Can you work these out from the model? Positions are in its coordinate system, mm. Face numbers are marked on the shaded views. Give positions to 0.01 mm unless a question says otherwise; leave off trailing zeros. Write each loop counter-clockwise with the first axis right and the second up, starting at its lowest first coordinate (ties: lowest second). Pieces come first, ordered by that corner, then holes.
from build123d import *

# Parameters (mm, degrees)
ESQUISSE1_R                  = 12
ESQUISSE1_R_2                = 10
BOSS_EXTRU_1_DEPTH           = 21
ESQUISSE2_R                  = 12
BOSS_EXTRU_2_DEPTH           = 24
ENL_V_MAT_EXTRU_1_DEPTH      = 49.093658626
ENL_V_MAT_EXTRU_1_DEPTH_BACK = 49.093658626
ENL_V_MAT_EXTRU_2_DEPTH      = 49.246865329
ENL_V_MAT_EXTRU_2_DEPTH_BACK = 49.246865329
ESQUISSE4_R                  = 1.65


with BuildPart() as part:
    # Esquisse1 → Boss.-Extru.1 (new body)
    with BuildSketch(Plane.XY):
        with Locations(Location((0, 0, 0), (0, 0, 180))):
            Circle(ESQUISSE1_R)
        with Locations(Location((0, 0, 0), (0, 0, 180))):
            Circle(ESQUISSE1_R_2, mode=Mode.SUBTRACT)
    extrude(amount=BOSS_EXTRU_1_DEPTH)

    # Esquisse2 → Boss.-Extru.2 (add)
    with BuildSketch(Plane.XY.offset(21)):
        with Locations(Location((0, 0, 0), (0, 0, 180))):
            Circle(ESQUISSE2_R)
    extrude(amount=BOSS_EXTRU_2_DEPTH)

    # Esquisse3 → Enlèv. mat.-Extru.1 (cut, two sides: drawn at the far end of the back side and taken through both)
    with BuildSketch(Plane(origin=(0, 0, 0), x_dir=(0, 0, -1), z_dir=(1, 0, 0)).offset(-ENL_V_MAT_EXTRU_1_DEPTH_BACK)):
        with BuildLine():
            Line((-33, 12), (-45, 12))
            Line((-45, 12), (-50, 0))
            Line((-50, 0), (-45, -12))
            Line((-45, -12), (-33, -12))
            ThreePointArc((-33, -12), (-45, 0), (-33, 12))
        make_face()
        with BuildLine():
            Line((-23.018016229, 0.6), (0, 0.6))
            Line((0, 0.6), (0, -0.6))
            Line((0, -0.6), (-23.018016229, -0.6))
            ThreePointArc((-23.018016229, -0.6), (-43, 0), (-23.018016229, 0.6))
        make_face()
    extrude(amount=ENL_V_MAT_EXTRU_1_DEPTH + ENL_V_MAT_EXTRU_1_DEPTH_BACK, mode=Mode.SUBTRACT)

    # Esquisse4 → Enlèv. mat.-Extru.2 (cut, two sides: drawn at the far end of the back side and taken through both)
    with BuildSketch(Plane(origin=(0, -0.6, 0), x_dir=(1, 0, 0), z_dir=(0, 1, 0)).offset(-ENL_V_MAT_EXTRU_2_DEPTH_BACK)):
        with Locations(Location((0, -16, 0), (0, 0, 270))):
            Circle(ESQUISSE4_R)
        with Locations(Location((0, -5, 0), (0, 0, 270))):
            Circle(ESQUISSE4_R)
    extrude(amount=ENL_V_MAT_EXTRU_2_DEPTH + ENL_V_MAT_EXTRU_2_DEPTH_BACK, mode=Mode.SUBTRACT)


solid = part.part
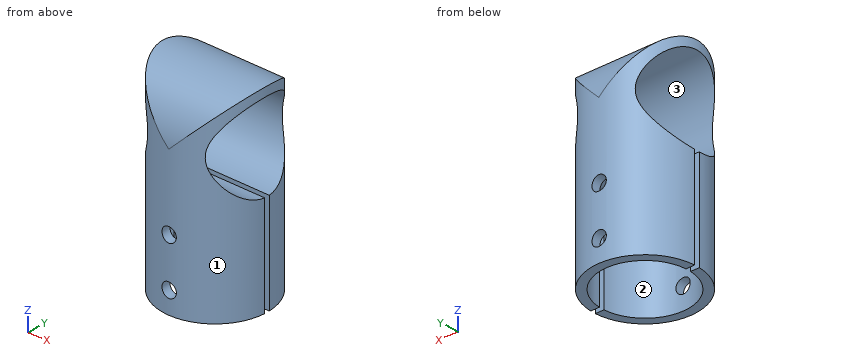
(1) Will these pins go through, and if not, where does the flat tip stop? P1, Ø5.5, axis at x = 0, z = 16, coming from the +Y side; P2, Ø4.5, axis at x = -2, y = -6, coming from the -Z side; P3, Ø1.5, axis at y = -7, z = 21.5, coming from the -X side; P4, Ø1, axis at x = 7, y = 5.5, coming from the +Z side.
Returned:
P1: stops at y = 12
P2: stops at z = 21
P3: stops at x = -10.24
P4: stops at z = 43.91
(2) If we mould it in two halves opening along X, with no side actions, what happens to the marked faces 1, 2 and 3? For each: +X half, -X half, draft (parallel to the pull), parting line (faces both ways), or undercut.
Returned:
face 1: parting line
face 2: undercut
face 3: draft
(3) Imagine slicing it at A-A, the plane x = 0. Write out the boundary of the cut face in (y, z).
Returned:
outline: (-12, 0) - (-10, 0) - (-10, 3.35) - (-12, 3.35) - close; (-12, 6.65) - (-10, 6.65) - (-10, 14.35) - (-12, 14.35) - close; (-12, 17.65) - (-10, 17.65) - (-10, 21) - (-0.6, 21) - (-0.6, 23.02) arc R10 cw (long way) to (0.6, 23.02) - (0.6, 21) - (10, 21) - (10, 17.65) - (12, 17.65) - (12, 33) arc R12 ccw to (-12, 33) - close; (10, 0) - (12, 0) - (12, 3.35) - (10, 3.35) - close; (10, 6.65) - (12, 6.65) - (12, 14.35) - (10, 14.35) - close
(4) Imagine slicing it at B-B, the plane y = 7.25. Write out the boundary of the cut face in (x, z), plus the area to 3 significant figures.
Returned:
outline: (-9.56, 0) - (-6.89, 0) - (-6.89, 21) - (6.89, 21) - (6.89, 0) - (9.56, 0) - (9.56, 26.11) - (-9.56, 26.11) - close; (-9.56, 39.89) - (9.56, 39.89) - (9.56, 42.56) - (-9.56, 42.56) - close
area: 261 mm2
(5) Imagine slicing it at C-C, the plane z = 16. Write out the boundary of the cut face in (x, y) (3 decimals).
Returned:
outline: (-11.985, -0.6) arc R12 ccw to (-1.65, -11.886) - (-1.65, -9.863) arc R10 cw to (-9.982, -0.6) - close; (-11.985, 0.6) - (-9.982, 0.6) arc R10 cw to (-1.65, 9.863) - (-1.65, 11.886) arc R12 ccw to start; (1.65, -11.886) arc R12 ccw to (11.985, -0.6) - (9.982, -0.6) arc R10 cw to (1.65, -9.863) - close; (1.65, 9.863) arc R10 cw to (9.982, 0.6) - (11.985, 0.6) arc R12 ccw to (1.65, 11.886) - close
(6) If I drill on L1, parallel to Z at x = -0.5, y = -10.75; L2, parallel to Z at x = 0, y = -11.05; L3, parallel to Z at x = 5, y = -5.5, over which ranges is the centre line in solid material (lowest first)?
Returned:
L1: z = 0 to 3.43, 6.57 to 14.43, 17.57 to 38.33
L2: z = 0 to 3.35, 6.65 to 14.35, 17.65 to 37.68
L3: z = 21 to 24.65, 41.35 to 43.67
(7) Imagine slicing it at D-D, the plane x = -9.25. Write out the boundary of the cut face in (y, z), plus the area to 3 significant figures.
Returned:
outline: (-7.64, 0) - (-3.8, 0) - (-3.8, 21) - (-0.6, 21) - (-0.6, 23.02) arc R10 cw to (-7.64, 26.55) - close; (-7.64, 39.45) arc R10 cw to (7.64, 39.45) - (7.64, 42.25) arc R12 ccw to (-7.64, 42.25) - close; (0.6, 21) - (3.8, 21) - (3.8, 0) - (7.64, 0) - (7.64, 26.55) arc R10 cw to (0.6, 23.02) - close
area: 240 mm2
